from build123d import *

# Parameters (mm, degrees)
SKETCH_1_R               = 9.25
SKETCH_1_R_2             = 2.5
EXTRUDE_1_DEPTH          = 7.5
SKETCH_3_R               = 1.75
CUT_EXTRUDE_1_DEPTH      = 13.25
CUT_EXTRUDE_1_DEPTH_BACK = 13.25
CHAMFER_1_SIZE           = 1
FILLET_1_R               = 2
CHAMFER_2_SIZE           = 1


with BuildPart() as part:
    # ｽｹｯﾁ1 → ﾎﾞｽ - 押し出し1 (new body, symmetric)
    with BuildSketch(Plane.XY):
        with BuildLine():
            Line((4, 12.25), (17.417201647, 4.809993282))
            ThreePointArc((17.417201647, 4.809993282), (20.25, 0), (17.417201647, -4.809993282))
            Line((17.417201647, -4.809993282), (4, -12.25))
            Line((4, -12.25), (-4, -12.25))
            Line((-4, -12.25), (-17.417201647, -4.809993282))
            ThreePointArc((-17.417201647, -4.809993282), (-20.25, 0), (-17.417201647, 4.809993282))
            Line((-17.417201647, 4.809993282), (-4, 12.25))
            Line((-4, 12.25), (4, 12.25))
        make_face()
        Circle(SKETCH_1_R, mode=Mode.SUBTRACT)
        with Locations((14.75, 0)):
            Circle(SKETCH_1_R_2, mode=Mode.SUBTRACT)
        with Locations((-14.75, 0)):
            Circle(SKETCH_1_R_2, mode=Mode.SUBTRACT)
    extrude(amount=EXTRUDE_1_DEPTH, both=True)

    # ｽｹｯﾁ3 → ｶｯﾄ - 押し出し1 (cut, two sides)
    with BuildSketch(Plane(origin=(0, 0, 0), x_dir=(1, 0, 0), z_dir=(0, 1, 0))) as cut_extrude_1_sk:
        Circle(SKETCH_3_R)
    extrude(amount=CUT_EXTRUDE_1_DEPTH, mode=Mode.SUBTRACT)
    extrude(cut_extrude_1_sk.sketch, amount=-CUT_EXTRUDE_1_DEPTH_BACK, mode=Mode.SUBTRACT)

    # 面取り1
    chamfer_1_edges = [part.edges().sort_by_distance(p)[0] for p in [
        (12.25, 0, -7.5),
        (12.25, 0, 7.5),
        (-17.25, 0, -7.5),
        (-17.25, 0, 7.5),
    ]]
    chamfer(chamfer_1_edges, length=CHAMFER_1_SIZE)

    # ﾌｨﾚｯﾄ1
    fillet_1_edges = [part.edges().sort_by_distance(p)[0] for p in [
        (4, -12.25, 0),
        (-4, -12.25, 0),
        (-4, 12.25, 0),
        (4, 12.25, 0),
    ]]
    fillet(fillet_1_edges, radius=FILLET_1_R)

    # 面取り2
    chamfer_2_edges = [part.edges().sort_by_distance(p)[0] for p in [
        (10.934845958, 8.404540874, -7.5),
        (20.25, 0, -7.5),
        (-20.25, 0, 7.5),
        (-10.934845958, -8.404540874, 7.5),
        (20.25, 0, 7.5),
        (10.934845958, -8.404540874, -7.5),
        (10.934845958, -8.404540874, 7.5),
        (0, -12.25, -7.5),
        (-10.934845958, 8.404540874, -7.5),
        (0, 12.25, -7.5),
        (-3.983509466, 12.186256302, -7.5),
        (3.983509466, 12.186256302, -7.5),
        (-3.983509466, -12.186256302, -7.5),
        (3.983509466, -12.186256302, -7.5),
        (0, -12.25, 7.5),
        (0, 12.25, 7.5),
        (-10.934845958, 8.404540874, 7.5),
        (-3.983509466, 12.186256302, 7.5),
        (3.983509466, 12.186256302, 7.5),
        (-3.983509466, -12.186256302, 7.5),
        (3.983509466, -12.186256302, 7.5),
        (10.934845958, 8.404540874, 7.5),
        (-10.934845958, -8.404540874, -7.5),
        (-20.25, 0, -7.5),
    ]]
    chamfer(chamfer_2_edges, length=CHAMFER_2_SIZE)


solid = part.part
Source: CAD feature listing. Evaluate the final solid. Frame: model axes, mm. Coordinates: 2 decimals unless noted, no trailing zeros. Loops run counter-clockwise (first coordinate to the right, second up) from the corner with the lowest first, then second, coordinate; pieces in that order, holes last. Notation, with made-up numbers: (-13.5, 27.25) - (-3.5, 27.25) arc R24 ccw to (-3.5, 46.25) - close; hole circle Ø4 at (50, 25.5). An arc over 180 degrees is marked (long way). Return JSON: item names as keys, results as strings.
Q1. Section C-C, the plane z = -2.5. Return loops of the section in (x, y), plus the area to 3 significant figures.
Results:
{"outline": "(-17.42, -4.81) - (-4.45, -12) arc R2 ccw to (-3.48, -12.25) - (3.48, -12.25) arc R2 ccw to (4.45, -12) - (17.42, -4.81) arc R5.5 ccw to (17.42, 4.81) - (4.45, 12) arc R2 ccw to (3.48, 12.25) - (-3.48, 12.25) arc R2 ccw to (-4.45, 12) - (-17.42, 4.81) arc R5.5 ccw to start; hole circle Ø5 at (-14.75, 0); hole circle Ø18.5 at (0, 0); hole circle Ø5 at (14.75, 0)", "area": "384 mm2"}
Q2. Section B-B, the plane y = 0. Return loops of the section in (x, z), plus the area to 3 significant figures.
Results:
{"outline": "(-20.25, -6.5) - (-19.25, -7.5) - (-18.25, -7.5) - (-17.25, -6.5) - (-17.25, 6.5) - (-18.25, 7.5) - (-19.25, 7.5) - (-20.25, 6.5) - close; (-12.25, -6.5) - (-11.25, -7.5) - (-9.25, -7.5) - (-9.25, 7.5) - (-11.25, 7.5) - (-12.25, 6.5) - close; (9.25, -7.5) - (11.25, -7.5) - (12.25, -6.5) - (12.25, 6.5) - (11.25, 7.5) - (9.25, 7.5) - close; (17.25, -6.5) - (18.25, -7.5) - (19.25, -7.5) - (20.25, -6.5) - (20.25, 6.5) - (19.25, 7.5) - (18.25, 7.5) - (17.25, 6.5) - close", "area": "174 mm2"}
Q3. Mould query, pull axis Y, two halves, no side actions, for faces 1 (the flat face through (0.05, -11.76, -6.99)), 2 (the cylindrical face through (-2.01, -9.03, -0.11)), 3 (the flat face through (10.844, 8.455, 0.091)). Classes: released by +Y, released by -Y, zero draft, split by the parting line, or undercut.
Results:
{"face 1": "released by -Y", "face 2": "undercut", "face 3": "released by +Y"}
Q4. Section D-D, the plane y = -8.25. Return loops of the section in (x, z), plus the area to 3 significant figures.
Results:
{"outline": "(-11.21, -6.5) - (-9.15, -7.5) - (-4.18, -7.5) - (-4.18, 7.5) - (-9.15, 7.5) - (-11.21, 6.5) - close; (4.18, -7.5) - (9.15, -7.5) - (11.21, -6.5) - (11.21, 6.5) - (9.15, 7.5) - (4.18, 7.5) - close", "area": "207 mm2"}
Q5. Material intervals for line 1 along Z through (x, y) = (0, -10.05); line 2 along X through (y, z) = (-0.25, 1.5); line 3 along Y through (x, z) = (0, -4), sorted ascending.
Results:
{"line 1": "-7.5 to -1.75, 1.75 to 7.5", "line 2": "-20.24 to -17.24, -12.26 to -9.25, 9.25 to 12.26, 17.24 to 20.24", "line 3": "-12.25 to -9.25, 9.25 to 12.25"}
Q6. Contact query for flat-ended pins moving along their axis: P1, Ø4, axis at x = 14.75, y = 0, coming from the -Z side; P2, Ø5, axis at x = -16, z = 2, coming from the -Y side; P3, Ø1, axis at y = -7, z = -3.5, coming from the -X side; P4, Ø6, axis at y = 8.5, z = -5.5, coming from the +X side. Output: stop coordinate, or through.
Results:
{"P1": "through", "P2": "y = -6.98", "P3": "x = -14.37", "P4": "x = 16.17"}
Q7. Section A-A, the plane z = 0. Return loops of the section in (x, y), plus the area to 3 significant figures.
Results:
{"outline": "(-17.42, -4.81) - (-4.45, -12) arc R2 ccw to (-3.48, -12.25) - (-1.75, -12.25) - (-1.75, -9.08) arc R9.25 cw to (-1.75, 9.08) - (-1.75, 12.25) - (-3.48, 12.25) arc R2 ccw to (-4.45, 12) - (-17.42, 4.81) arc R5.5 ccw to start; (1.75, -12.25) - (3.48, -12.25) arc R2 ccw to (4.45, -12) - (17.42, -4.81) arc R5.5 ccw to (17.42, 4.81) - (4.45, 12) arc R2 ccw to (3.48, 12.25) - (1.75, 12.25) - (1.75, 9.08) arc R9.25 cw to (1.75, -9.08) - close; hole circle Ø5 at (-14.75, 0); hole circle Ø5 at (14.75, 0)", "area": "363 mm2"}
